```python
from build123d import *

# Parameters (mm, degrees)
F0_R     = 50
F1_DEPTH = 2.5
F2_R     = 2.5
F3_DEPTH = 12
F4_SIZE  = 1


with BuildPart() as f1:
    # F0 (on Right) → F1 (new body, symmetric)
    with BuildSketch(Plane.YZ):
        Circle(F0_R)
        with BuildLine():
            ThreePointArc((2.5, 44.930501889), (26.4503363532, 36.4057647469), (41.958904116, 16.2619299402))
            ThreePointArc((41.958904116, 16.2619299402), (42.7975432333, 13.9057647469), (43.5039890879, 11.5066473588))
            ThreePointArc((43.5039890879, 11.5066473588), (44.6244300185, 5.8017450411), (45, 0))
            ThreePointArc((45, 0), (40.6475171403, -19.3074946672), (28.4320288744, -34.8800764633))
            ThreePointArc((28.4320288744, -34.8800764633), (26.4503363532, -36.4057647469), (24.3869439025, -37.8190027248))
            ThreePointArc((24.3869439025, -37.8190027248), (0, -45), (-24.3869439025, -37.8190027248))
            ThreePointArc((-24.3869439025, -37.8190027248), (-26.4503363532, -36.4057647469), (-28.4320288744, -34.8800764633))
            ThreePointArc((-28.4320288744, -34.8800764633), (-42.7975432333, -13.9057647469), (-43.5039890879, 11.5066473588))
            ThreePointArc((-43.5039890879, 11.5066473588), (-42.7975432333, 13.9057647469), (-41.958904116, 16.2619299402))
            ThreePointArc((-41.958904116, 16.2619299402), (-26.4503363532, 36.4057647469), (-2.5, 44.930501889))
            ThreePointArc((-2.5, 44.930501889), (0, 45), (2.5, 44.930501889))
        make_face(mode=Mode.SUBTRACT)
        with BuildLine():
            ThreePointArc((-2.5, 4.3301270189), (0, 5), (2.5, 4.3301270189))
            Line((2.5, 4.3301270189), (2.5, 44.930501889))
            ThreePointArc((2.5, 44.930501889), (0, 45), (-2.5, 44.930501889))
            Line((-2.5, 44.930501889), (-2.5, 4.3301270189))
        make_face()
        with BuildLine():
            ThreePointArc((-4.8907380037, -1.0395584541), (-4.7552825815, 1.5450849719), (-3.3456530318, 3.7157241274))
            Line((-3.3456530318, 3.7157241274), (-41.958904116, 16.2619299402))
            ThreePointArc((-41.958904116, 16.2619299402), (-42.7975432333, 13.9057647469), (-43.5039890879, 11.5066473588))
            Line((-43.5039890879, 11.5066473588), (-4.8907380037, -1.0395584541))
        make_face()
        with BuildLine():
            Line((-24.3869439025, -37.8190027248), (-0.5226423163, -4.9726094768))
            ThreePointArc((-0.5226423163, -4.9726094768), (-2.9389262615, -4.0450849719), (-4.5677272882, -2.0336832154))
            Line((-4.5677272882, -2.0336832154), (-28.4320288744, -34.8800764633))
            ThreePointArc((-28.4320288744, -34.8800764633), (-26.4503363532, -36.4057647469), (-24.3869439025, -37.8190027248))
        make_face()
        with BuildLine():
            Line((28.4320288744, -34.8800764633), (4.5677272882, -2.0336832154))
            ThreePointArc((4.5677272882, -2.0336832154), (2.9389262615, -4.0450849719), (0.5226423163, -4.9726094768))
            Line((0.5226423163, -4.9726094768), (24.3869439025, -37.8190027248))
            ThreePointArc((24.3869439025, -37.8190027248), (26.4503363532, -36.4057647469), (28.4320288744, -34.8800764633))
        make_face()
        with BuildLine():
            ThreePointArc((3.3456530318, 3.7157241274), (4.5677272882, 2.0336832154), (5, 0))
            ThreePointArc((5, 0), (4.9726094768, -0.5226423163), (4.8907380037, -1.0395584541))
            Line((4.8907380037, -1.0395584541), (43.5039890879, 11.5066473588))
            ThreePointArc((43.5039890879, 11.5066473588), (42.7975432333, 13.9057647469), (41.958904116, 16.2619299402))
            Line((41.958904116, 16.2619299402), (3.3456530318, 3.7157241274))
        make_face()
        Polygon((2.5, 0.8122992406), (2.5, 3.4409548012), (0, 2.6286555606), (-2.5, 3.4409548012), (-2.5, 0.8122992406), (-4.0450849719, -1.3143277803), (-1.5450849719, -2.1266270209), (0, -4.2532540418), (1.5450849719, -2.1266270209), (4.0450849719, -1.3143277803), align=None)
        with BuildLine():
            Line((2.5, 3.4409548012), (2.5, 4.3301270189))
            ThreePointArc((2.5, 4.3301270189), (0, 5), (-2.5, 4.3301270189))
            Line((-2.5, 4.3301270189), (-2.5, 3.4409548012))
            Line((-2.5, 3.4409548012), (0, 2.6286555606))
            Line((0, 2.6286555606), (2.5, 3.4409548012))
        make_face()
        with BuildLine():
            Line((-2.5, 3.4409548012), (-3.3456530318, 3.7157241274))
            ThreePointArc((-3.3456530318, 3.7157241274), (-4.7552825815, 1.5450849719), (-4.8907380037, -1.0395584541))
            Line((-4.8907380037, -1.0395584541), (-4.0450849719, -1.3143277803))
            Line((-4.0450849719, -1.3143277803), (-2.5, 0.8122992406))
            Line((-2.5, 0.8122992406), (-2.5, 3.4409548012))
        make_face()
        with BuildLine():
            ThreePointArc((-4.5677272882, -2.0336832154), (-2.9389262615, -4.0450849719), (-0.5226423163, -4.9726094768))
            Line((-0.5226423163, -4.9726094768), (0, -4.2532540418))
            Line((0, -4.2532540418), (-1.5450849719, -2.1266270209))
            Line((-1.5450849719, -2.1266270209), (-4.0450849719, -1.3143277803))
            Line((-4.0450849719, -1.3143277803), (-4.5677272882, -2.0336832154))
        make_face()
        with BuildLine():
            ThreePointArc((0.5226423163, -4.9726094768), (2.9389262615, -4.0450849719), (4.5677272882, -2.0336832154))
            Line((4.5677272882, -2.0336832154), (4.0450849719, -1.3143277803))
            Line((4.0450849719, -1.3143277803), (1.5450849719, -2.1266270209))
            Line((1.5450849719, -2.1266270209), (0, -4.2532540418))
            Line((0, -4.2532540418), (0.5226423163, -4.9726094768))
        make_face()
        with BuildLine():
            ThreePointArc((4.8907380037, -1.0395584541), (4.9726094768, -0.5226423163), (5, 0))
            ThreePointArc((5, 0), (4.5677272882, 2.0336832154), (3.3456530318, 3.7157241274))
            Line((3.3456530318, 3.7157241274), (2.5, 3.4409548012))
            Line((2.5, 3.4409548012), (2.5, 0.8122992406))
            Line((2.5, 0.8122992406), (4.0450849719, -1.3143277803))
            Line((4.0450849719, -1.3143277803), (4.8907380037, -1.0395584541))
        make_face()
    extrude(amount=F1_DEPTH, both=True)

    # F2 (on face) → F3 (join)
    with BuildSketch(Plane.YZ.offset(2.5)):
        Circle(F2_R)
    extrude(amount=F3_DEPTH)

    # F4
    f4_edges = [f1.edges().sort_by_distance(p)[0] for p in [
        (14.5, -2.5, 0),
    ]]
    chamfer(f4_edges, length=F4_SIZE)


solid = f1.part
```
Source: CAD feature listing. Evaluate the final solid. Frame: model axes, mm. A direction names the side the tool comes from. Round coordinates to 2 decimals unless told otherwise and drop trailing zeros. Loops run counter-clockwise (first coordinate to the right, second up) from the corner with the lowest first, then second, coordinate; pieces in that order, holes last.
1. Section query C-C on y = -15. Output: boundary loops of the cut face in (x, z), and give its area (3 significant figures).
2. Mould query, pull axis Y, two halves, no side actions, for faces 1 (the flat face through (14.5, 0, 0)), 2 (the cylindrical face through (0.04, 47.69, 15.02)), 3 (the cylindrical face through (0.035, 26.158, 36.617)), 4 (the flat face through (0, 2.5, 24)). Classes: released by +Y, released by -Y, zero draft, split by the parting line, or undercut.
3. Access query for faces 5 (the cylindrical face through (0.04, 42.91, -13.56)), 6 (the cylindrical face through (7.92, -0.54, -2.44)), 7 (the flat face through (-2.5, 0, 0)). Directions: +Z, -Z, +X, -X, +Y, -Y. A direction counts if a zero-diameter tool reaches every point of the face in a straight line with its end or side. Return the directions, or none.
4. Section query A-A on x = 0.5. Output: boundary loops of the cut face in (y, z), and give its area (3 significant figures).
5. Section query D-D on z = 22. Output: boundary loops of the cut face in (x, y).
6. Ray query, L1, parallel to Y at x = 0.25, z = 35; L2, parallel to Z at x = -1.5, y = 32; L3, parallel to Z at x = 0.25, y = -30. Return the intervals inside material, ascending.
7. Section query B-B on z = -14.5. Output: boundary loops of the cut face in (x, y).
8. Contact query for flat-ended pins moving along their axis: pin 1 (5 mm diameter, centred on x = 8, z = 0.5, fed in from +Y); pin 2 (6 mm diameter, centred on x = 3, y = 5, fed in from -Z); pin 3 (2 mm diameter, centred on x = 1, y = -13, fed in from +Z). Output: stop coordinate, or through.
Answers below:
1. outline: (-2.5, -47.7) - (2.5, -47.7) - (2.5, -42.43) - (-2.5, -42.43) - close; (-2.5, -24.9) - (2.5, -24.9) - (2.5, -16.39) - (-2.5, -16.39) - close; (-2.5, 2.25) - (2.5, 2.25) - (2.5, 7.5) - (-2.5, 7.5) - close; (-2.5, 42.43) - (2.5, 42.43) - (2.5, 47.7) - (-2.5, 47.7) - close
1. area: 122 mm2
2. face 1: zero draft
2. face 2: split by the parting line
2. face 3: undercut
2. face 4: undercut
3. face 5: +X, -X
3. face 6: +X
3. face 7: +Z, -Z, -X, +Y, -Y
4. outline: circle Ø100 at (0, 0); hole (-43.5, 11.51) arc R45 ccw to (-28.43, -34.88) - (-4.05, -1.31) - close; hole (-41.96, 16.26) - (-2.5, 3.44) - (-2.5, 44.93) arc R45 ccw to start; hole (-24.39, -37.82) arc R45 ccw to (24.39, -37.82) - (0, -4.25) - close; hole (2.5, 3.44) - (41.96, 16.26) arc R45 ccw to (2.5, 44.93) - close; hole (4.05, -1.31) - (28.43, -34.88) arc R45 ccw to (43.5, 11.51) - close
4. area: 2,570 mm2
5. outline: (-2.5, -44.9) - (2.5, -44.9) - (2.5, -39.26) - (-2.5, -39.26) - close; (-2.5, -2.5) - (2.5, -2.5) - (2.5, 2.5) - (-2.5, 2.5) - close; (-2.5, 39.26) - (2.5, 39.26) - (2.5, 44.9) - (-2.5, 44.9) - close
6. L1: y = -35.71 to -28.28, -2.5 to 2.5, 28.28 to 35.71
6. L2: z = -38.42 to -31.64, 7.77 to 13.03, 31.64 to 38.42
6. L3: z = -40 to -33.54, 7.12 to 12.38, 33.54 to 40
7. outline: (-2.5, -47.85) - (2.5, -47.85) - (2.5, -42.6) - (-2.5, -42.6) - close; (-2.5, -13.63) - (2.5, -13.63) - (2.5, -7.44) - (-2.5, -7.44) - close; (-2.5, 7.44) - (2.5, 7.44) - (2.5, 13.63) - (-2.5, 13.63) - close; (-2.5, 42.6) - (2.5, 42.6) - (2.5, 47.85) - (-2.5, 47.85) - close
8. pin 1: stops at y = 2.5
8. pin 2: stops at z = -49.96
8. pin 3: stops at z = 48.54
